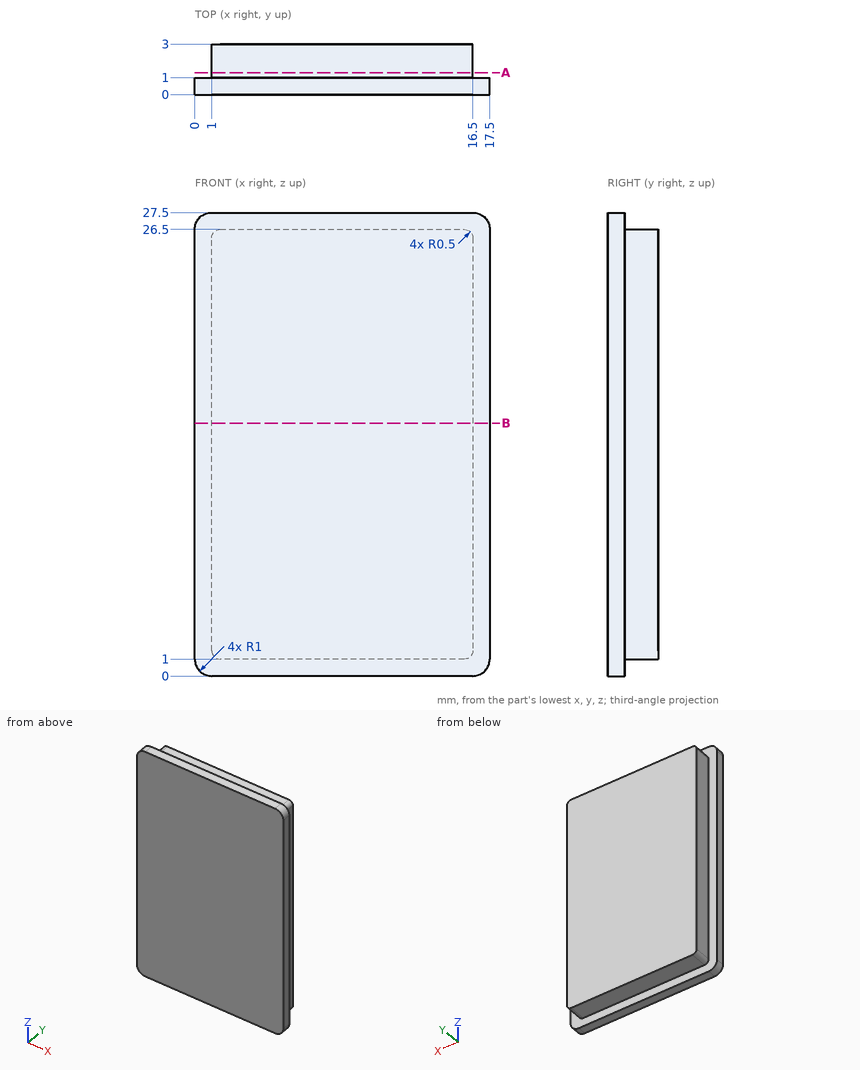
Job drawing, mm, ordinate dimensions from the low corner. One solid piece. Give positions to 0.01 mm unless a question says otherwise; leave off trailing zeros. Loops run counter-clockwise (first coordinate to the right, second up) from the corner with the lowest first, then second, coordinate; pieces in that order, holes last. Notation, with made-up numbers: M 3,-33 L 8,-33 A18 cw 8,-29 Z; hole C 20,82 d6. An arc over 180 degrees is marked long. Return JSON: item names as keys, results as strings.
1) Flat gauge pins, fed straight in: pin 1 Ø1.6 at (x, y) = (5, 2.5) entering from +Z; pin 2 Ø1.5 at (x, y) = (12, 1.5) entering from -Z; pin 3 Ø0.6 at (y, z) = (1.5, 19.5) entering from +X; pin 4 Ø1.6 at (y, z) = (2.5, 19) entering from -X. Where does each tip first touch, or does it go through?
Calculated:
{"pin 1": "stops at z = 26.5", "pin 2": "stops at z = 0", "pin 3": "stops at x = 16.5", "pin 4": "stops at x = 1"}
2) Drill centre lines: line 1 (X direction, y = 2.05, z = 16); line 2 (Z direction, x = 5.5, y = 2.2); line 3 (Z direction, x = 16.75, y = 0.3). Where is each one in solid material? Low to high.
Calculated:
{"line 1": "x = 1 to 16.5", "line 2": "z = 1 to 26.5", "line 3": "z = 0.03 to 27.47"}
3) Saw through at B-B, the plane z = 15. List the corners of the cut face in (x, y), then the cut area to 3 significant figures.
Calculated:
{"outline": "M 0,0 L 17.5,0 L 17.5,1 L 16.5,1 L 16.5,3 L 1,3 L 1,1 L 0,1 Z", "area": "48.5 mm2"}
4) Saw through at A-A, the plane y = 1.3. List the corners of the cut face in (x, z), then the cut area to 3 significant figures.
Calculated:
{"outline": "M 1,1.5 A0.5 ccw 1.5,1 L 16,1 A0.5 ccw 16.5,1.5 L 16.5,26 A0.5 ccw 16,26.5 L 1.5,26.5 A0.5 ccw 1,26 Z", "area": "395 mm2"}
